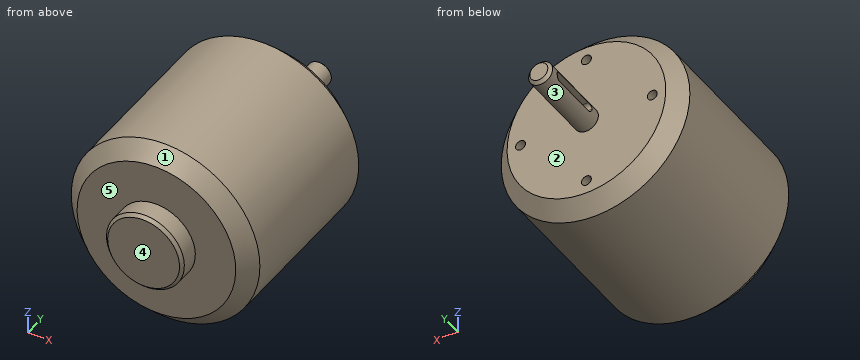
```python
from build123d import *

# Parameters (mm, degrees)
SKETCH1_R               = 31.5
BOSS_EXTRUDE1_DEPTH     = 64
SKETCH2_R               = 4
BOSS_EXTRUDE2_DEPTH     = 26
CHAMFER3_SIZE           = 1
CUT_EXTRUDE1_REACH      = 102.422
CUT_EXTRUDE1_END_RADIUS = 4
SKETCH3_W               = 3
SKETCH3_H               = 19
FILLET1_R               = 1.5
CIRPATTERN2_COUNT       = 4
CHAMFER4_SIZE           = 5
SKETCH11_R              = 13
BOSS_EXTRUDE3_DEPTH     = 7
CHAMFER5_SIZE           = 1


with BuildPart() as part:
    # Sketch1 → Boss-Extrude1 (new body)
    with BuildSketch(Plane(origin=(0, 0, 0), x_dir=(1, 0, 0), z_dir=(0, 1, 0))):
        with Locations(Location((0, 0, 0), (0, 0, 270))):
            Circle(SKETCH1_R)
    extrude(amount=BOSS_EXTRUDE1_DEPTH)

    # Sketch2 → Boss-Extrude2 (add)
    with BuildSketch(Plane(origin=(0, 64, 0), x_dir=(1, 0, 0), z_dir=(0, 1, 0))):
        with Locations(Location((0, 0, 0), (0, 0, 90))):
            Circle(SKETCH2_R)
    extrude(amount=BOSS_EXTRUDE2_DEPTH)

    # Chamfer3
    chamfer3_edges = [part.edges().sort_by_distance(p)[0] for p in [
        (0, 90, 4),
    ]]
    chamfer(chamfer3_edges, length=CHAMFER3_SIZE)

    # Cut-Extrude1: up to this cylinder (the profile starts inside it)
    cut_extrude1_end = Plane(origin=(0, 77, 0), z_dir=(0, -1, 0)) * Cylinder(CUT_EXTRUDE1_END_RADIUS, 213.844, mode=Mode.PRIVATE)
    # Sketch3 → Cut-Extrude1 (cut, up to the surface)
    with BuildSketch(Plane(origin=(0, 0, 0), x_dir=(0, 0, -1), z_dir=(1, 0, 0)), mode=Mode.PRIVATE) as cut_extrude1_sk1:
        with Locations((0, 77)):
            Rectangle(SKETCH3_W, SKETCH3_H)
    cut_extrude1_tool1 = extrude(cut_extrude1_sk1.sketch, amount=-CUT_EXTRUDE1_REACH, mode=Mode.PRIVATE) & cut_extrude1_end
    add(cut_extrude1_tool1.solids().sort_by_distance((0, 77, 0))[0], mode=Mode.SUBTRACT)

    # Fillet1
    fillet1_edges = [part.edges().sort_by_distance(p)[0] for p in [
        (-1.854049622, 67.5, -1.5),
        (-1.854049622, 67.5, 1.5),
        (-1.854049622, 86.5, -1.5),
        (-1.854049622, 86.5, 1.5),
    ]]
    fillet(fillet1_edges, radius=FILLET1_R - 0.0001)  # a hair under: the kernel refuses the full size

    # Sketch10 → M4 Tapped Hole1 (revolve, cut)
    with BuildSketch(Plane(origin=(0, 64, -22), x_dir=(0, 0, 1), z_dir=(1, 0, 0))):
        Polygon((0, 0), (0, 13.091420021), (1.65, 12.1), (1.65, 0), align=None)
    m4_tapped_hole1 = revolve(axis=Axis((0, 70.35, -22), (0, -1, 0)), mode=Mode.SUBTRACT)

    # CirPattern2: M4 Tapped Hole1 ×4 about axis
    cirpattern2_axis = Axis((0, 0, 0), (0, 1, 0))
    for i in range(1, CIRPATTERN2_COUNT):
        add(m4_tapped_hole1.rotate(cirpattern2_axis, i * 360 / CIRPATTERN2_COUNT), mode=Mode.SUBTRACT)

    # Chamfer4
    chamfer4_edges = [part.edges().sort_by_distance(p)[0] for p in [
        (0, 0, -31.5),
        (0, 64, -31.5),
    ]]
    chamfer(chamfer4_edges, length=CHAMFER4_SIZE)

    # Sketch11 → Boss-Extrude3 (add)
    with BuildSketch(Plane(origin=(0, 0, 0), x_dir=(-1, 0, 0), z_dir=(0, -1, 0))):
        with Locations(Location((0, 0, 0), (0, 0, 270))):
            Circle(SKETCH11_R)
    extrude(amount=BOSS_EXTRUDE3_DEPTH)

    # Chamfer5
    chamfer5_edges = [part.edges().sort_by_distance(p)[0] for p in [
        (0, -7, -13),
    ]]
    chamfer(chamfer5_edges, length=CHAMFER5_SIZE)


solid = part.part
```
For this review, take the finished solid that the model builds, in its own axes (mm). Face numbers are marked on the shaded views. A direction names the side the tool comes from. Give positions to 0.01 mm unless a question says otherwise; leave off trailing zeros. Order: outer loops, then holes, each group sorted by start corner. A loop starts at its lowest first (then second) coordinate and runs counter-clockwise, first axis right, second up.
1) The part is to be moulded in two halves that separate along X. For the marked faces 1 and 2, say which applies: released by +X, released by -X, zero draft, split by the parting line, or undercut.
2) For the marked faces 3, 4 and 5, list the 3-axis set-ups (+Z, -Z, +X, -X, +Y, -Y) from which the entire face can be reached by the end or side of a thin tool; tool diameter is ignored.
3) Wall thickness on line 1 (Z direction, x = -22, y = 56); line 2 (Y direction, x = -21.5, z = -14.5): over which ranges is each line inside the solid? List them lowest first.
4) Take a section at A-A (y = 43). Give the boundary of the cut face in (x, z).
5) Insertion check: pin 1 (5.5 mm diameter, centred on x = 0, z = 22, fed in from -Y); pin 2 (8 mm diameter, centred on x = 25, y = 69.5, fed in from -Z) (3 decimals); pin 3 (4 mm diameter, centred on x = -14.5, y = 25.5, fed in from -Z); pin 4 (8 mm diameter, centred on y = 13.5, z = 19, fed in from +X). Each pin has a flat end and moves straight along its axis. Give the tip position at first contact, or say it passes through.
Derived:
1. face 1: split by the parting line
1. face 2: zero draft
2. face 3: +Y
2. face 4: +Z, -Z, +X, -X, -Y
2. face 5: -Y
3. line 1: z = -22.54 to -1.65, 1.65 to 22.54
3. line 2: y = 0 to 64
4. outline: circle Ø63 at (0, 0)
5. pin 1: stops at y = 0
5. pin 2: passes through
5. pin 3: stops at z = -28.91
5. pin 4: stops at x = 27.7
